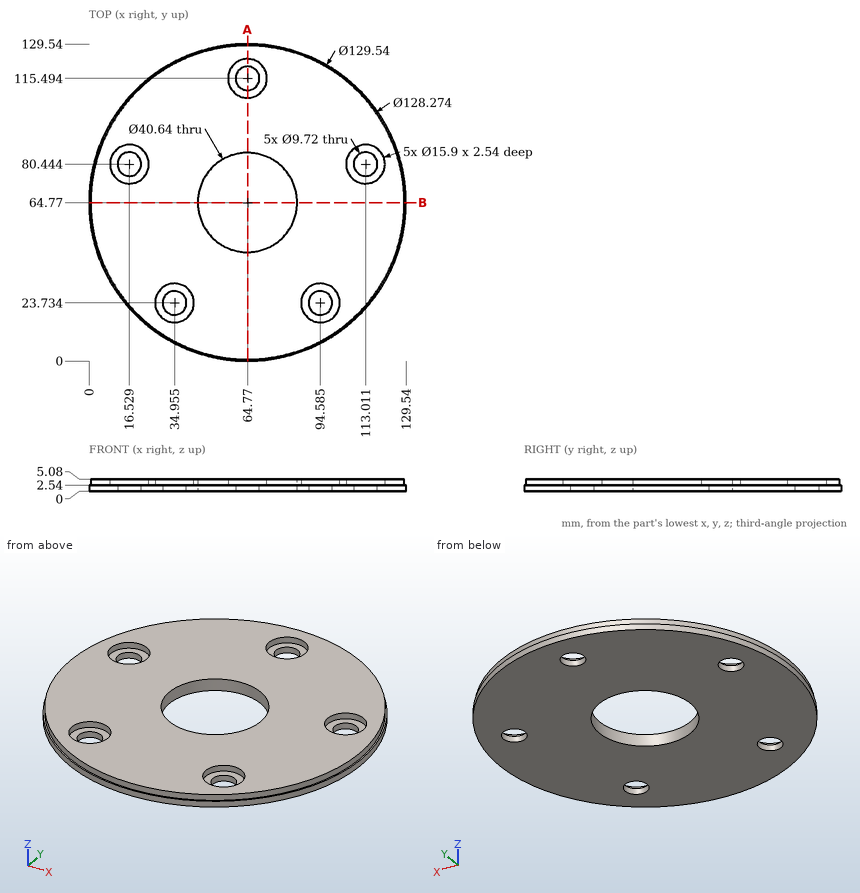
Could you check a few things on this drawing? It's one solid part, dimensions in mm from its lowest x, y, z. Coordinates: 2 decimals unless noted, no trailing zeros. Write each loop counter-clockwise with the first axis right and the second up, starting at its lowest first coordinate (ties: lowest second). Pieces come first, ordered by that corner, then holes.
1) If we section it at A-A (x = 64.77): Count the separate pieces of the cut face and the enclosed holes in it.
Filled in:
separate pieces: 3
enclosed holes: 0
2) I'm going to push flat-ended pins straight in: pin 1 (5 mm diameter, centred on x = 33.5, y = 27, fed in from +Z); pin 2 (1.5 mm diameter, centred on x = 64.5, z = 2, fed in from -Y); pin 3 (1.5 mm diameter, centred on y = 19, z = 2.5, fed in from +X) (1 decimal). Where does each tip first touch, or does it pass through?
Filled in:
pin 1: stops at z = 2.54
pin 2: stops at y = 0
pin 3: stops at x = 111.3
3) If we section it at B-B (y = 64.77): List the corners of the cut face in (x, z) for me.
Filled in:
outline: (0, 0) - (44.45, 0) - (44.45, 5.08) - (0.63, 5.08) - (0.63, 2.54) - (0, 2.54) - close; (85.09, 0) - (129.54, 0) - (129.54, 2.54) - (128.91, 2.54) - (128.91, 5.08) - (85.09, 5.08) - close
4) If I drill on line 1 (Y direction, x = 67, z = 4.2) (1 decimal); line 2 (Y direction, x = 65.5, z = 1.95) (1 decimal); line 3 (Y direction, x = 31, z = 1.4) (1 decimal), over which ranges is the centre line in solid material (lowest first)?
Filled in:
line 1: y = 0.7 to 44.6, 85 to 107.9, 123.1 to 128.9
line 2: y = 0 to 44.5, 85.1 to 110.7, 120.3 to 129.5
line 3: y = 9.5 to 20.9, 26.6 to 120
